Could you check a few things on this model? Use its own coordinates, in mm. Face numbers are marked on the shaded views. A direction names the side the tool comes from. Round coordinates to 2 decimals unless told otherwise and drop trailing zeros. Write each question's results on one line, items separated by ' | '. Start each with the question number.
1) We'd pull the mould along Z, two halves only. Please class the marked faces 1, 2, 3 and 4: pulls with the +Z half, pulls with the -Z half, needs draft (parallel to the pull), parting line crosses it, or undercut.
2) If I drill on probe 1 along Z at (x, y) = (0, 6); probe 2 along X at (y, z) = (-3.75, 4); probe 3 along Z at (x, y) = (0, 12.95), over which ranges is the centre line in solid material (lowest first)?
3) Which directions (+Z, -Z, +X, -X, +Y, -Y) give clear straight access to the entire face, cutting with the end or side of a thin tool? Please do the marked faces 5 and 6.
4) For P1, Ø2.5, axis at x = 0, z = 34.3, coming from the -Y side; P2, Ø10, axis at x = 10, z = 33, coming from the -Y side; P3, Ø0.6, axis at x = -0.5, z = 7, coming from the -Y side, each with a flat end and sliding along its axis, tell me the tip position at first contact or that it passes through.
5) Imagine slicing it at A-A, the plane y = 10.25. Give the number of separate pieces and of enclosed holes in the cut face, plus the area to 3 significant figures.
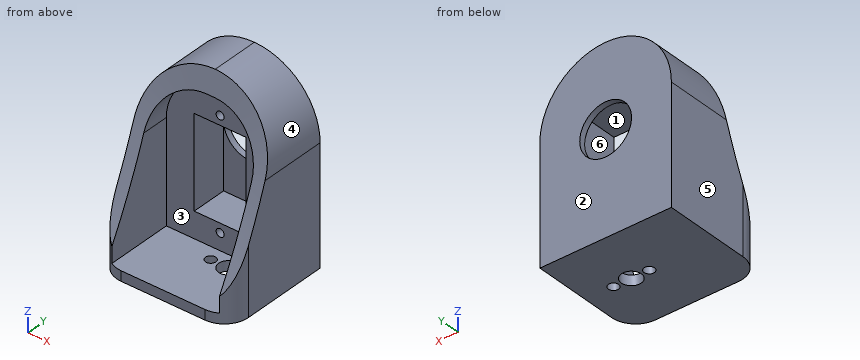
from build123d import *

# Parameters (mm, degrees)
SKETCH1_W           = 33
SKETCH1_H           = 28
BOSS_EXTRUDE1_DEPTH = 46
CUT_EXTRUDE1_DEPTH  = 59.318093247
CUT_EXTRUDE2_START  = -3
CUT_EXTRUDE2_DEPTH  = 27
FILLET1_R           = 12.5
FILLET2_R           = 16.5
FILLET3_R           = 6
SKETCH5_W           = 13
SKETCH5_H           = 23
CUT_EXTRUDE3_DEPTH  = 9
SKETCH6_R           = 6.5
CUT_EXTRUDE5_DEPTH  = 56.592265809
SKETCH7_R           = 1
CUT_EXTRUDE6_DEPTH  = 8
SKETCH8_R           = 1.3
SKETCH8_R_2         = 2.5
CUT_EXTRUDE7_DEPTH  = 2.5


with BuildPart() as part:
    # Sketch1 → Boss-Extrude1 (new body)
    with BuildSketch(Plane.XY):
        Rectangle(SKETCH1_W, SKETCH1_H)
    extrude(amount=BOSS_EXTRUDE1_DEPTH)

    # Sketch3 → Cut-Extrude1 (cut, through all)
    with BuildSketch(Plane(origin=(16.5, 0, 0), x_dir=(0, 0, -1), z_dir=(1, 0, 0))):
        with BuildLine():
            Line((-5, -14), (-46, -14))
            Line((-46, -14), (-46, 2))
            add(Edge.make_bspline(
                [(-46, 2), (-24.590873565, -3.089136006), (-5, -14)],
                knots=[0, 0, 0, 1, 1, 1], degree=2))
        make_face()
    extrude(amount=-CUT_EXTRUDE1_DEPTH, mode=Mode.SUBTRACT)

    # Sketch4 → Cut-Extrude2 (cut)
    with BuildSketch(Plane(origin=(16.5, 0, 0), x_dir=(0, 0, -1), z_dir=(1, 0, 0)).offset(CUT_EXTRUDE2_START)):
        with BuildLine():
            Line((-5, -14), (-2.5, -14))
            Line((-2.5, -14), (-2.5, 3.5))
            Line((-2.5, 3.5), (-40.5, 3.5))
            Line((-40.5, 3.5), (-40.5, 0.588274649))
            add(Edge.make_bspline(
                [(-5, -14), (-22.060550055, -4.498364419), (-40.5, 0.588274649)],
                knots=[0, 0, 0, 1, 1, 1], degree=2))
        make_face()
    extrude(amount=-CUT_EXTRUDE2_DEPTH, mode=Mode.SUBTRACT)

    # Fillet1
    fillet1_edges = [part.edges().sort_by_distance(p)[0] for p in [
        (13.5, 2.044137325, 40.5),
        (-13.5, 2.044137325, 40.5),
    ]]
    fillet(fillet1_edges, radius=FILLET1_R)

    # Fillet2
    fillet2_edges = [part.edges().sort_by_distance(p)[0] for p in [
        (16.5, 8, 46),
        (-16.5, 8, 46),
    ]]
    fillet(fillet2_edges, radius=FILLET2_R - 0.0001)  # a hair under: the kernel refuses the full size

    # Fillet3
    fillet3_edges = [part.edges().sort_by_distance(p)[0] for p in [
        (-16.5, -14, 2.5),
        (16.5, -14, 2.5),
    ]]
    fillet(fillet3_edges, radius=FILLET3_R)

    # Sketch5 → Cut-Extrude3 (cut)
    with BuildSketch(Plane.XZ.offset(-3.5)):
        with Locations((0, 20.5)):
            Rectangle(SKETCH5_W, SKETCH5_H)
    extrude(amount=-CUT_EXTRUDE3_DEPTH, mode=Mode.SUBTRACT)

    # Sketch6 → Cut-Extrude5 (cut, through all)
    with BuildSketch(Plane.XZ.offset(-12.5)):
        with Locations((0, 25.5)):
            Circle(SKETCH6_R)
    extrude(amount=-CUT_EXTRUDE5_DEPTH, mode=Mode.SUBTRACT)

    # Sketch7 → Cut-Extrude6 (cut)
    with BuildSketch(Plane.XZ.offset(-3.5)):
        with Locations((0, 34.3)):
            Circle(SKETCH7_R)
        with Locations((0, 6.7)):
            Circle(SKETCH7_R)
    extrude(amount=-CUT_EXTRUDE6_DEPTH, mode=Mode.SUBTRACT)

    # Sketch8 → Cut-Extrude7 (cut)
    with BuildSketch(Plane(origin=(0, 0, 0), x_dir=(-1, 0, 0), z_dir=(0, 0, -1))):
        with Locations((-9.5, 0)):
            Circle(SKETCH8_R)
        with Locations((-5, 0)):
            Circle(SKETCH8_R_2)
        with Locations((-0.5, 0)):
            Circle(SKETCH8_R)
    extrude(amount=-CUT_EXTRUDE7_DEPTH, mode=Mode.SUBTRACT)


solid = part.part
Checked values:
1) face 1: undercut | face 2: needs draft | face 3: undercut | face 4: pulls with the +Z half
2) probe 1: 0 to 5.7, 7.7 to 9, 32 to 33.3, 35.3 to 46 | probe 2: -16.5 to -13.5, 13.5 to 16.5 | probe 3: 0 to 19, 32 to 46
3) face 5: +Z, -Z, -X, +Y, -Y | face 6: -Y
4) P1: y = 3.5 | P2: y = -2.93 | P3: y = 11.5
5) separate pieces: 1 | enclosed holes: 3 | area: 1,100 mm^2
